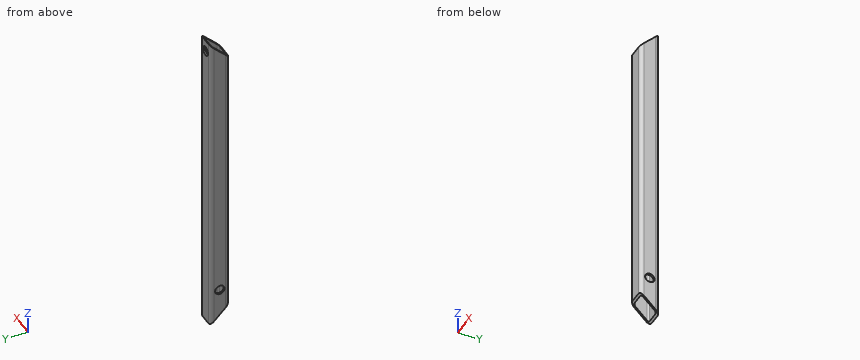
Autodesk Inventor part; units mm, degrees
ref_plane "Piano iniziale" through (0, 0, 0) normal (0, 0, 1) x (1, 0, 0)
ref_plane "Piano finale" through (0, 0, 340) normal (0, 0, 1) x (1, 0, 0)
ref_plane "YZ Plane" through (0, 0, 0) normal (1, 0, 0) x (0, 1, 0)
ref_plane "Piano iniziale" through (0, 0, 0) normal (0, 0, 1) x (1, 0, 0)
ref_plane "Piano finale" through (0, 0, 340) normal (0, 0, 1) x (1, 0, 0)
sketch "Schizzo" plane through (0, 0, 0) normal (0, 0, 1) x (1, 0, 0)
  line L0 (-10, -6) -> (-10, 6)
  line L1 (-6, 10) -> (6, 10)
  line L2 (10, 6) -> (10, -6)
  line L3 (6, -10) -> (-6, -10)
  arc A0 (-10, -6) -> (-6, -10) centre (-6, -6) ccw
  arc A1 (10, 6) -> (6, 10) centre (6, 6) ccw
  arc A2 (-6, 10) -> (-10, 6) centre (-6, 6) ccw
  arc A3 (6, -10) -> (10, -6) centre (6, -6) ccw
  arc A4 (-6, 8) -> (-8, 6) centre (-6, 6) ccw
  line L4 (-6, 8) -> (6, 8)
  arc A5 (8, 6) -> (6, 8) centre (6, 6) ccw
  line L5 (8, 6) -> (8, -6)
  arc A6 (6, -8) -> (8, -6) centre (6, -6) ccw
  line L6 (6, -8) -> (-6, -8)
  arc A7 (-8, -6) -> (-6, -8) centre (-6, -6) ccw
  line L7 (-8, -6) -> (-8, 6)
  line L8 (0, 15.1598) -> (0, -15.1598) construction
  line L9 (-15.1598, 0) -> (15.1598, 0) construction
  dimension "d7" = 4
  dimension "d9" = 20
  dimension "d11" = 20
  dimension "d12" = 2
  dimension "d15" = 10
  dimension "d16" = 10
extrude "Corpo" add sketch "Schizzo" along normal up to surface (340 mm away) from surface at 0
sketch "Sketch3" plane through (0, 0, 0) normal (0, 0, 1) x (1, 0, 0)
  line L0 (0, 0) -> (10, 0)
ref_plane "Work Plane3" through (0, 0, 0) normal (0, -1, 0) x (1, 0, 0)
sketch "Sketch4" plane through (0, 0, 0) normal (0, -1, 0) x (1, 0, 0)
  line L0 (-2, 0) -> (12, 0)
  line L1 (-2, 340) -> (12, 340)
  dimension "d18" = 340
sketch "Schizzo5" plane through (-10, 6, 0) normal (-1, 0, 0) x (0, 0, 1)
  line L0 (0, 4) -> (0, 0)
  line L1 (0, 4) -> (28.5929, -24.5929)
  line L2 (0, 4) -> (40.4365, 4) construction
  line L3 (28.5929, -24.5929) -> (0, -24.5929)
  line L4 (0, -24.5929) -> (0, 4)
  line L5 (340, 4) -> (340, 0)
  line L6 (340, 4) -> (307.9608, -28.0392)
  line L7 (340, 4) -> (385.3103, 4) construction
  line L8 (307.9608, -28.0392) -> (340, -28.0392)
  line L9 (340, -28.0392) -> (340, 4)
  line L10 (340, 0) -> (340, -12)
  point P0 (0, -6)
  dimension "d19" = 45
  dimension "d20" = 135
extrude "Estrusione2" cut sketch "Schizzo5" against normal up to next
sketch "Schizzo6" plane through (6, 10, 340) normal (0, 1, 0) x (1, 0, 0)
  line L0 (-12, 0) -> (0, 0)
  point P0 (-6, 340)
  point P1 (-6, 12.5)
  point P2 (-6, 0)
  dimension "d23" = 12.5
hole "Foro1" at (0, 10, 327.5) direction (0, -1, 0) diameter 10 depth 5 tip angle 118
sketch "Schizzo7" plane through (-10, 6, 4) normal (-1, 0, 0) x (0, 0, 1)
  point P0 (-4, -6)
  point P1 (36, -6)
  dimension "d31" = 40
hole "Foro2" at (-10, 0, 40) direction (1, 0, 0) diameter 10 end through all
equation "\"d7\" = G_IR"
equation "\"d9\" = G_W"
equation "\"d11\" = G_H"
equation "\"d12\" = G_T"
equation "\"d15\" = 0.5 * d9"
equation "\"d16\" = 0.5 * d11"
equation "\"d3\" = G_L"
equation "\"G_W\" = 20"
equation "\"G_H\" = 20"
equation "\"G_T\" = 2"
equation "\"G_IR\" = 4"
equation "\"G_L\" = d18"
equation "\"G_OFFSET_START\" = 0"
equation "\"G_OFFSET_END\" = 0"
properties part number "ISO 10799-2 - 20x20x2 - 340" material "Acciaio, Dolce"
Input: part model. Units: mm. Frame: model coordinates. Give positions to 0.01 mm unless a question says otherwise; leave off trailing zeros. Loops run counter-clockwise (first coordinate to the right, second up) from the corner with the lowest first, then second, coordinate; pieces in that order, holes last.
1) Section query C-C on z = 202. Return the cut outline in (x, y).
A:
outline: (-10, -6) arc R4 ccw to (-6, -10) - (6, -10) arc R4 ccw to (10, -6) - (10, 6) arc R4 ccw to (6, 10) - (-6, 10) arc R4 ccw to (-10, 6) - close; hole (-8, -6) arc R2 ccw to (-6, -8) - (6, -8) arc R2 ccw to (8, -6) - (8, 6) arc R2 ccw to (6, 8) - (-6, 8) arc R2 ccw to (-8, 6) - close
2) Line query: L1, parallel to X at y = -1.25, z = 236.5; L2, parallel to Z at x = 0, y = 9.25. Output: solid intervals per line, ascending.
A:
L1: x = -10 to -8, 8 to 10
L2: z = 0.75 to 322.5, 332.5 to 339.25
3) Section query D-D on z = 40. Return the cut outline in (x, y), and give its area (3 significant figures).
A:
outline: (-10, -6) arc R4 ccw to (-6, -10) - (6, -10) arc R4 ccw to (10, -6) - (10, -5) - (8, -5) - (8, -6) arc R2 cw to (6, -8) - (-6, -8) arc R2 cw to (-8, -6) - (-8, -5) - (-10, -5) - close; (-10, 5) - (-8, 5) - (-8, 6) arc R2 cw to (-6, 8) - (6, 8) arc R2 cw to (8, 6) - (8, 5) - (10, 5) - (10, 6) arc R4 ccw to (6, 10) - (-6, 10) arc R4 ccw to (-10, 6) - close
area: 93.7 mm2
4) Section query A-A on z = 327.5. Return the cut outline in (x, y), and give its area (3 significant figures).
A:
outline: (-10, -2.5) - (-8, -2.5) - (-8, 6) arc R2 cw to (-6, 8) - (-5, 8) - (-5, 10) - (-6, 10) arc R4 ccw to (-10, 6) - close; (5, 8) - (6, 8) arc R2 cw to (8, 6) - (8, -2.5) - (10, -2.5) - (10, 6) arc R4 ccw to (6, 10) - (5, 10) - close
area: 56.8 mm2
5) Section query B-B on x = 0. Return the cut outline in (y, z), and give its area (3 significant figures).
A:
outline: (-10, 20) - (-8, 18) - (-8, 322) - (-10, 320) - close; (8, 2) - (10, 0) - (10, 322.5) - (8, 322.5) - close; (8, 332.5) - (10, 332.5) - (10, 340) - (8, 338) - close
area: 1,260 mm2
6) Contact query for flat-ended pins moving along their axis: pin 1 (2 mm diameter, centred on x = 6, y = -3.5, fed in from -Z); pin 2 (12 mm diameter, centred on x = -3, y = 2.5, fed in from -Z). Output: stop coordinate, or through.
A:
pin 1: passes through
pin 2: stops at z = 1.5
